```python
from build123d import *

# Parameters (mm, degrees)
SKETCH_1_R          = 51.5
EXTRUDE_1_DEPTH     = 4
SKETCH_2_R          = 54
EXTRUDE_2_DEPTH     = 4
SKETCH_3_R          = 29.5
CUT_EXTRUDE_1_DEPTH = 10
SKETCH_4_R          = 3
CUT_EXTRUDE_2_DEPTH = 10
CHAMFER_2_SIZE      = 2.5
SKETCH_5_R          = 2
CUT_EXTRUDE_3_DEPTH = 10


with BuildPart() as part:
    # Эскиз1 → Бобышка-Вытянуть1 (new body)
    with BuildSketch(Plane(origin=(0, 0, 0), x_dir=(1, 0, 0), z_dir=(0, 1, 0))):
        with Locations(Location((0, 0, 0), (0, 0, 270))):
            Circle(SKETCH_1_R)
    extrude(amount=EXTRUDE_1_DEPTH)

    # Эскиз2 → Бобышка-Вытянуть2 (add)
    with BuildSketch(Plane(origin=(0, 4, 0), x_dir=(1, 0, 0), z_dir=(0, 1, 0))):
        with Locations(Location((0, 0, 0), (0, 0, 270))):
            Circle(SKETCH_2_R)
    extrude(amount=EXTRUDE_2_DEPTH)

    # Эскиз3 → Вырез-Вытянуть1 (cut)
    with BuildSketch(Plane(origin=(0, 8, 0), x_dir=(1, 0, 0), z_dir=(0, 1, 0))):
        with Locations(Location((0, 0, 0), (0, 0, 270))):
            Circle(SKETCH_3_R)
    extrude(amount=-CUT_EXTRUDE_1_DEPTH, mode=Mode.SUBTRACT)

    # Эскиз4 → Вырез-Вытянуть2 (cut)
    with BuildSketch(Plane(origin=(0, 8, 0), x_dir=(1, 0, 0), z_dir=(0, 1, 0))):
        with Locations(Location((0, 42.5, 0), (0, 0, 270))):
            Circle(SKETCH_4_R)
        with Locations(Location((-42.5, 0, 0), (0, 0, 270))):
            Circle(SKETCH_4_R)
        with Locations(Location((0, -42.5, 0), (0, 0, 270))):
            Circle(SKETCH_4_R)
        with Locations(Location((42.5, 0, 0), (0, 0, 270))):
            Circle(SKETCH_4_R)
    extrude(amount=-CUT_EXTRUDE_2_DEPTH, mode=Mode.SUBTRACT)

    # Фаска2
    chamfer_2_edges = [part.edges().sort_by_distance(p)[0] for p in [
        (0, 8, -45.5),
        (-42.5, 8, -3),
        (0, 8, 39.5),
        (42.5, 8, -3),
    ]]
    chamfer(chamfer_2_edges, length=CHAMFER_2_SIZE)

    # Эскиз5 → Вырез-Вытянуть3 (cut)
    with BuildSketch(Plane(origin=(0, 8, 0), x_dir=(1, 0, 0), z_dir=(0, 1, 0))):
        with Locations(Location((30.0520382, -30.0520382, 0), (0, 0, 270))):
            Circle(SKETCH_5_R)
    extrude(amount=-CUT_EXTRUDE_3_DEPTH, mode=Mode.SUBTRACT)


solid = part.part
```
Part model, mm, in its own coordinate system. A direction names the side the tool comes from. Round coordinates to 2 decimals unless told otherwise and drop trailing zeros. Loops run counter-clockwise (first coordinate to the right, second up) from the corner with the lowest first, then second, coordinate; pieces in that order, holes last. Notation, with made-up numbers: (45, 50.5) -> (78, 50.5) arc R10 cw to (78, 63.5) -> close; hole circle Ø5 at (-12.5, -24.75). An arc over 180 degrees is marked (long way). Use a Markdown table: item, result.
1) Probe line 1 (X direction, y = 3.25, z = 0); line 2 (X direction, y = 5.25, z = 0); line 3 (Z direction, x = -2.5, y = 7). List the from-to ranges inside material, lowest first. Write a range as [from, to].
The answers:
| item | result |
|---|---|
| line 1 | x = [-51.5, -45.5], [-39.5, -29.5], [29.5, 39.5], [45.5, 51.5] |
| line 2 | x = [-54, -45.5], [-39.5, -29.5], [29.5, 39.5], [45.5, 54] |
| line 3 | z = [-53.94, -46.24], [-38.76, -29.39], [29.39, 38.76], [46.24, 53.94] |
2) Drop flat-ended pins along their axis: pin 1 Ø1 at (x, y) = (34, 4) entering from +Z; pin 2 Ø5 at (x, z) = (42.5, 0) entering from +Y; pin 3 Ø2 at (x, y) = (10.5, 2.5) entering from +Z; pin 4 Ø3 at (x, y) = (7.5, 4) entering from +Z. Give the stop position or say it passes through.
The answers:
| item | result |
|---|---|
| pin 1 | stops at z = 42.35 |
| pin 2 | passes through |
| pin 3 | stops at z = 50.62 |
| pin 4 | stops at z = 53.67 |
3) Pull direction X, two halves, no side cores. Call faces 1 (the flat face through (-23, 8, 23)), 2 (the cylindrical face through (0.1, 2.8, -45.5)), 3 (the cylindrical face through (-45.69, 1.97, 23.76)): pulls with the +X half, pulls with the -X half, needs draft (parallel to the pull), parting line crosses it, or undercut.
The answers:
| item | result |
|---|---|
| face 1 | needs draft |
| face 2 | undercut |
| face 3 | parting line crosses it |
4) Cut at C-C, the plane y = 6.75. List the corners of the cut face in (x, z), and give its area (3 significant figures).
The answers:
| item | result |
|---|---|
| outline | circle Ø108 at (0, 0); hole circle Ø8.5 at (-42.5, 0); hole circle Ø59 at (0, 0); hole circle Ø8.5 at (0, -42.5); hole circle Ø8.5 at (0, 42.5); hole circle Ø4 at (30.05, 30.05); hole circle Ø8.5 at (42.5, 0) |
| area | 6,190 mm2 |
5) Cut at A-A, the plane z = 0. List the corners of the cut face in (x, y).
The answers:
| item | result |
|---|---|
| outline | (-54, 4) -> (-51.5, 4) -> (-51.5, 0) -> (-45.5, 0) -> (-45.5, 5.5) -> (-48, 8) -> (-54, 8) -> close; (-39.5, 0) -> (-29.5, 0) -> (-29.5, 8) -> (-37, 8) -> (-39.5, 5.5) -> close; (29.5, 0) -> (39.5, 0) -> (39.5, 5.5) -> (37, 8) -> (29.5, 8) -> close; (45.5, 0) -> (51.5, 0) -> (51.5, 4) -> (54, 4) -> (54, 8) -> (48, 8) -> (45.5, 5.5) -> close |
6) Tool access for faces 4 (the cylindrical face through (0.1, 2.8, 39.5)), 5 (the flat face through (-20, 4, 48)): list every direction of +Z, -Z, +X, -X, +Y, -Y with a clear straight run to the whole face (end or side of a thin tool).
The answers:
| item | result |
|---|---|
| face 4 | +Y, -Y |
| face 5 | -Y |
7) Cut at D-D, the plane x = 17. List the corners of the cut face in (y, z).
The answers:
| item | result |
|---|---|
| outline | (0, -48.61) -> (4, -48.61) -> (4, -51.25) -> (8, -51.25) -> (8, -24.11) -> (0, -24.11) -> close; (0, 24.11) -> (8, 24.11) -> (8, 51.25) -> (4, 51.25) -> (4, 48.61) -> (0, 48.61) -> close |
8) Cut at B-B, the plane x = 0. List the corners of the cut face in (y, z).
The answers:
| item | result |
|---|---|
| outline | (0, -51.5) -> (4, -51.5) -> (4, -54) -> (8, -54) -> (8, -48) -> (5.5, -45.5) -> (0, -45.5) -> close; (0, -39.5) -> (5.5, -39.5) -> (8, -37) -> (8, -29.5) -> (0, -29.5) -> close; (0, 29.5) -> (8, 29.5) -> (8, 37) -> (5.5, 39.5) -> (0, 39.5) -> close; (0, 45.5) -> (5.5, 45.5) -> (8, 48) -> (8, 54) -> (4, 54) -> (4, 51.5) -> (0, 51.5) -> close |
